from build123d import *

# Parameters (mm, degrees)
SKETCH1_W           = 33.528
SKETCH1_H           = 20.066
BOSS_EXTRUDE1_DEPTH = 3.556
SKETCH2_W           = 28.448
SKETCH2_H           = 14.986
CUT_EXTRUDE1_DEPTH  = 2.72199989
CUT_EXTRUDE2_REACH  = 37.177
SKETCH3_W           = 8.599089176
SKETCH3_H           = 2.434237831
CUT_EXTRUDE3_REACH  = 37.177
FILLET1_R           = 1.524
FILLET2_R           = 0.508
FILLET3_R           = 1.27
SKETCH7_R           = 0.911071032
CUT_EXTRUDE4_DEPTH  = 1.27
SKETCH9_R           = 0.530860858
CUT_EXTRUDE5_DEPTH  = 20.857943524
FILLET4_R           = 0.254
FILLET5_R           = 0.254


with BuildPart() as part:
    # Sketch1 → Boss-Extrude1 (new body)
    with BuildSketch(Plane(origin=(0, 0, 0), x_dir=(1, 0, 0), z_dir=(0, 1, 0))):
        Rectangle(SKETCH1_W, SKETCH1_H)
    extrude(amount=BOSS_EXTRUDE1_DEPTH)

    # Sketch2 → Cut-Extrude1 (cut)
    with BuildSketch(Plane(origin=(0, 3.556, 0), x_dir=(1, 0, 0), z_dir=(0, 1, 0))):
        Rectangle(SKETCH2_W, SKETCH2_H)
    extrude(amount=-CUT_EXTRUDE1_DEPTH, mode=Mode.SUBTRACT)

    # Sketch3 → Cut-Extrude2 (cut, up to next)
    with BuildSketch(Plane(origin=(16.764, 0, 0), x_dir=(0, 0, -1), z_dir=(1, 0, 0)), mode=Mode.PRIVATE) as cut_extrude2_sk1:
        with Locations((0, 2.338881085)):
            Rectangle(SKETCH3_W, SKETCH3_H)
    cut_extrude2_tool1 = extrude(cut_extrude2_sk1.sketch, amount=-CUT_EXTRUDE2_REACH, mode=Mode.PRIVATE) & part.part
    add(cut_extrude2_tool1.solids().sort_by_distance((16.764, 2.338881, 0))[0], mode=Mode.SUBTRACT)

    # Sketch5 → Cut-Extrude3 (cut, up to next)
    with BuildSketch(Plane.ZY.offset(16.764), mode=Mode.PRIVATE) as cut_extrude3_sk1:
        Polygon((-3.991394218, 3.556), (3.991394218, 3.556), (3.484543993, 1.607179709), (-3.484543993, 1.607179709), align=None)
    cut_extrude3_tool1 = extrude(cut_extrude3_sk1.sketch, amount=-CUT_EXTRUDE3_REACH, mode=Mode.PRIVATE) & part.part
    add(cut_extrude3_tool1.solids().sort_by_distance((-16.764, 2.603611, 0))[0], mode=Mode.SUBTRACT)

    # Fillet1
    fillet1_edges = [part.edges().sort_by_distance(p)[0] for p in [
        (-15.494, 1.607179709, -3.484543993),
        (-15.494, 1.607179709, 3.484543993),
    ]]
    fillet(fillet1_edges, radius=FILLET1_R)

    # Fillet2
    fillet2_edges = [part.edges().sort_by_distance(p)[0] for p in [
        (15.494, 1.121762169, 4.299544588),
        (15.494, 1.121762169, -4.299544588),
    ]]
    fillet(fillet2_edges, radius=FILLET2_R)

    # Fillet3
    fillet3_edges = [part.edges().sort_by_distance(p)[0] for p in [
        (16.764, 1.778, 10.033),
        (-16.764, 1.778, 10.033),
        (-16.764, 1.778, -10.033),
        (16.764, 1.778, -10.033),
    ]]
    fillet(fillet3_edges, radius=FILLET3_R)

    # Sketch7 → Cut-Extrude4 (cut)
    with BuildSketch(Plane.XZ):
        with Locations(Location((-14.683903523, 8.287062989, 0), (0, 0, 270))):
            Circle(SKETCH7_R)
        with Locations(Location((14.683903523, 8.287062989, 0), (0, 0, 270))):
            Circle(SKETCH7_R)
        with Locations(Location((14.683903523, -8.287062989, 0), (0, 0, 270))):
            Circle(SKETCH7_R)
        with Locations(Location((-14.683903523, -8.287062989, 0), (0, 0, 270))):
            Circle(SKETCH7_R)
    extrude(amount=-CUT_EXTRUDE4_DEPTH, mode=Mode.SUBTRACT)

    # Sketch9 → Cut-Extrude5 (cut, through all)
    with BuildSketch(Plane.XZ):
        with Locations(Location((-14.683903523, 8.287062989, 0), (0, 0, 270))):
            Circle(SKETCH9_R)
        with Locations(Location((14.683903523, 8.287062989, 0), (0, 0, 270))):
            Circle(SKETCH9_R)
        with Locations(Location((14.683903523, -8.287062989, 0), (0, 0, 270))):
            Circle(SKETCH9_R)
        with Locations(Location((-14.683903523, -8.287062989, 0), (0, 0, 270))):
            Circle(SKETCH9_R)
    extrude(amount=-CUT_EXTRUDE5_DEPTH, mode=Mode.SUBTRACT)

    # Fillet4
    fillet4_edges = [part.edges().sort_by_distance(p)[0] for p in [
        (14.224, 2.195000055, -7.493),
        (14.224, 2.195000055, 7.493),
        (-14.224, 2.195000055, 7.493),
        (-14.224, 2.195000055, -7.493),
    ]]
    fillet(fillet4_edges, radius=FILLET4_R)

    # Fillet5
    fillet5_edges = [part.edges().sort_by_distance(p)[0] for p in [
        (14.224, 0.83400011, 0),
        (0, 0.83400011, 7.493),
        (0, 0.83400011, -7.493),
        (-14.224, 0.83400011, 0),
        (-14.149605122, 0.83400011, -7.418605122),
        (14.149605122, 0.83400011, -7.418605122),
        (-14.149605122, 0.83400011, 7.418605122),
        (14.149605122, 0.83400011, 7.418605122),
    ]]
    fillet(fillet5_edges, radius=FILLET5_R)


solid = part.part
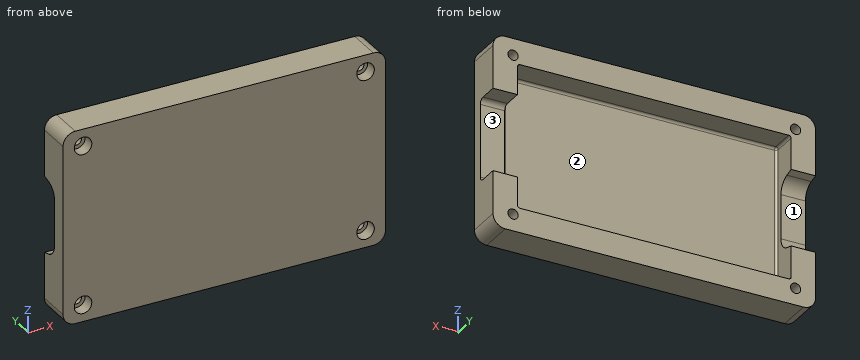
Can you work these out from the model? Positions are in its coordinate system, mm. Face numbers are marked on the shaded views. A direction names the side the tool comes from. Round coordinates to 2 decimals unless told otherwise and drop trailing zeros. Loops run counter-clockwise (first coordinate to the right, second up) from the corner with the lowest first, then second, coordinate; pieces in that order, holes last. Notation, with made-up numbers: (-7, 51) - (27, 51) arc R33 ccw to (27, 89) - close; hole circle Ø2 at (70, 53.25). An arc over 180 degrees is marked (long way). Use CSV: the item, a comma, the result in double quotes. Start each with the question number.
1) Please list where these lines run through material, in increasing order: probe 1 along Z at (x, y) = (-6.5, 2.3); probe 2 along X at (y, z) = (2, -6.75); probe 3 along X at (y, z) = (1.15, 8). Write a range as [from, to].
2) If we section it at D-D on y = 0.35: Write out the boundary of the cut face in (x, z).
3) If we section it at C-C on x = -0.5: Write out the boundary of the cut face in (y, z), plus the area to 3 significant figures.
4) If we section it at B-B on z = -6.25: Write out the boundary of the cut face in (x, y).
5) For pin 1 Ø1.5 at (x, z) = (14.68, 8.29) entering from -Y; pin 2 Ø1.3 at (x, z) = (-16, -1) entering from +Y, each with a flat end and sliding along its axis, tell me the tip position at first contact or that it passes through.
6) For the marked faces 1, 2 and 3, which set-ups out of +Z, -Z, +X, -X, +Y, -Y let a thin tool reach every point of the face, with its end or its side?
7) If we section it at A-A on y = 1.95: Write out the boundary of the cut face in (x, z).
Geometry results:
1,probe 1,"z = [-10.03, -7.49], [7.49, 10.03]"
1,probe 2,"x = [-16.76, -14.22], [14.22, 16.76]"
1,probe 3,"x = [-16.76, -15.55], [-13.82, 13.82], [15.55, 16.76]"
2,outline,"(-16.76, -8.76) arc R1.27 ccw to (-15.49, -10.03) - (15.49, -10.03) arc R1.27 ccw to (16.76, -8.76) - (16.76, 8.76) arc R1.27 ccw to (15.49, 10.03) - (-15.49, 10.03) arc R1.27 ccw to (-16.76, 8.76) - close; hole circle Ø1.82 at (-14.68, -8.29); hole circle Ø1.82 at (-14.68, 8.29); hole circle Ø1.82 at (14.68, -8.29); hole circle Ø1.82 at (14.68, 8.29)"
3,outline,"(0, -10.03) - (3.56, -10.03) - (3.56, -7.49) - (1.09, -7.49) arc R0.25 cw to (0.83, -7.24) - (0.83, 7.24) arc R0.25 cw to (1.09, 7.49) - (3.56, 7.49) - (3.56, 10.03) - (0, 10.03) - close"
3,area,"30.6 mm2"
4,outline,"(-16.76, 0) - (16.76, 0) - (16.76, 3.56) - (14.22, 3.56) - (14.22, 1.09) arc R0.25 cw to (13.97, 0.83) - (-13.97, 0.83) arc R0.25 cw to (-14.22, 1.09) - (-14.22, 3.56) - (-16.76, 3.56) - close"
5,pin 1,"stops at y = 1.27"
5,pin 2,"stops at y = 1.61"
6,face 1,"+X, -X, +Y"
6,face 2,"+Y"
6,face 3,"+X, +Y"
7,outline,"(-16.76, -8.76) arc R1.27 ccw to (-15.49, -10.03) - (15.49, -10.03) arc R1.27 ccw to (16.76, -8.76) - (16.76, -4.3) - (14.22, -4.3) - (14.22, -7.24) arc R0.25 cw to (13.97, -7.49) - (-13.97, -7.49) arc R0.25 cw to (-14.22, -7.24) - (-14.22, -3.27) - (-16.76, -3.27) - close; (-16.76, 3.27) - (-14.22, 3.27) - (-14.22, 7.24) arc R0.25 cw to (-13.97, 7.49) - (13.97, 7.49) arc R0.25 cw to (14.22, 7.24) - (14.22, 4.3) - (16.76, 4.3) - (16.76, 8.76) arc R1.27 ccw to (15.49, 10.03) - (-15.49, 10.03) arc R1.27 ccw to (-16.76, 8.76) - close; hole circle Ø1.06 at (-14.68, -8.29); hole circle Ø1.06 at (-14.68, 8.29); hole circle Ø1.06 at (14.68, -8.29); hole circle Ø1.06 at (14.68, 8.29)"
